Read the model definition and answer for the solid it produces. Units are mm, in the model's axes. Coordinates: 2 decimals unless noted, no trailing zeros. Loops run counter-clockwise (first coordinate to the right, second up) from the corner with the lowest first, then second, coordinate; pieces in that order, holes last.
Q1. Straight lines are drawn through the part: line 1 (X direction, y = 0.4, z = 0); line 2 (X direction, y = 0.3, z = -3); line 3 (Z direction, x = 2, y = 0.8). For each, find the intervals that lie inside material, in ascending order.
Q2. Section B-B (z = 3.75) is taken. Give the vertices of the cut face in (x, y), then the cut area to 3 significant figures.
Q3. A flat-ended cylindrical pin translates along its axis: P1, Ø0.7, axis at x = 0, z = 0, coming from the +Y side. Find the tip coordinate at first contact, or state that the pin passes through.
Q4. Section C-C (x = -3.75) is taken. Give the vertices of the cut face in (y, z).
Q5. Section D-D (y = 0.85) is taken. Count the separate pieces of the cut face and the enclosed holes in it, then the cut area to 3 significant figures.
Q6. Section A-A (x = 0) is taken. Give the vertices of the cut face in (y, z), then the cut area to 3 significant figures.
Q7. The mould has two halves that part along Z. Classify faces 1 (the face through (2.285, 0.493, -3.584)), 2 (the face through (0.525, 0.493, -0.165)), 3 (the face through (0, 1, 1)): pulls with the +Z half, pulls with the -Z half, needs draft (parallel to the pull), parting line crosses it, or undercut.
from build123d import *

# Parameters (mm, degrees)
ESQUISSE1_R        = 4.25
ESQUISSE1_R_2      = 0.55
ESQUISSE1_R_3      = 0.2
ESQUISSE1_R_4      = 0.3
BOSS_EXTRU_2_DEPTH = 1


with BuildPart() as part:
    # Esquisse1 → Boss.-Extru.2 (new body)
    with BuildSketch(Plane(origin=(0, 0, 0), x_dir=(1, 0, 0), z_dir=(0, 1, 0))):
        Circle(ESQUISSE1_R)
        Circle(ESQUISSE1_R_2, mode=Mode.SUBTRACT)
        with Locations((0, 3)):
            Circle(ESQUISSE1_R_3, mode=Mode.SUBTRACT)
        with Locations((0, 3.75)):
            Circle(ESQUISSE1_R_4, mode=Mode.SUBTRACT)
        with Locations((0.717946993, 2.912825452)):
            Circle(ESQUISSE1_R_3, mode=Mode.SUBTRACT)
        with Locations((1.394169516, 2.656368077)):
            Circle(ESQUISSE1_R_3, mode=Mode.SUBTRACT)
        with Locations((1.989367975, 2.245532245)):
            Circle(ESQUISSE1_R_3, mode=Mode.SUBTRACT)
        with Locations((2.468951598, 1.70419424)):
            Circle(ESQUISSE1_R_3, mode=Mode.SUBTRACT)
        with Locations((2.805048728, 1.063814661)):
            Circle(ESQUISSE1_R_3, mode=Mode.SUBTRACT)
        with Locations((2.978126622, 0.361610041)):
            Circle(ESQUISSE1_R_3, mode=Mode.SUBTRACT)
        with Locations((2.978126622, -0.361610041)):
            Circle(ESQUISSE1_R_3, mode=Mode.SUBTRACT)
        with Locations((2.805048728, -1.063814661)):
            Circle(ESQUISSE1_R_3, mode=Mode.SUBTRACT)
        with Locations((2.468951598, -1.70419424)):
            Circle(ESQUISSE1_R_3, mode=Mode.SUBTRACT)
        with Locations((1.989367975, -2.245532245)):
            Circle(ESQUISSE1_R_3, mode=Mode.SUBTRACT)
        with Locations((1.394169516, -2.656368077)):
            Circle(ESQUISSE1_R_3, mode=Mode.SUBTRACT)
        with Locations((0.717946993, -2.912825452)):
            Circle(ESQUISSE1_R_3, mode=Mode.SUBTRACT)
        with Locations((0, -3)):
            Circle(ESQUISSE1_R_3, mode=Mode.SUBTRACT)
        with Locations((-0.717946993, -2.912825452)):
            Circle(ESQUISSE1_R_3, mode=Mode.SUBTRACT)
        with Locations((-1.394169516, -2.656368077)):
            Circle(ESQUISSE1_R_3, mode=Mode.SUBTRACT)
        with Locations((-1.989367975, -2.245532245)):
            Circle(ESQUISSE1_R_3, mode=Mode.SUBTRACT)
        with Locations((-2.468951598, -1.70419424)):
            Circle(ESQUISSE1_R_3, mode=Mode.SUBTRACT)
        with Locations((-2.805048728, -1.063814661)):
            Circle(ESQUISSE1_R_3, mode=Mode.SUBTRACT)
        with Locations((-2.978126622, -0.361610041)):
            Circle(ESQUISSE1_R_3, mode=Mode.SUBTRACT)
        with Locations((-2.978126622, 0.361610041)):
            Circle(ESQUISSE1_R_3, mode=Mode.SUBTRACT)
        with Locations((-2.805048728, 1.063814661)):
            Circle(ESQUISSE1_R_3, mode=Mode.SUBTRACT)
        with Locations((-2.468951598, 1.70419424)):
            Circle(ESQUISSE1_R_3, mode=Mode.SUBTRACT)
        with Locations((-1.989367975, 2.245532245)):
            Circle(ESQUISSE1_R_3, mode=Mode.SUBTRACT)
        with Locations((-1.394169516, 2.656368077)):
            Circle(ESQUISSE1_R_3, mode=Mode.SUBTRACT)
        with Locations((-0.717946993, 2.912825452)):
            Circle(ESQUISSE1_R_3, mode=Mode.SUBTRACT)
        with Locations((3.75, 0)):
            Circle(ESQUISSE1_R_4, mode=Mode.SUBTRACT)
        with Locations((0, -3.75)):
            Circle(ESQUISSE1_R_4, mode=Mode.SUBTRACT)
        with Locations((-3.75, 0)):
            Circle(ESQUISSE1_R_4, mode=Mode.SUBTRACT)
    extrude(amount=BOSS_EXTRU_2_DEPTH)


solid = part.part
Numbers:
1. line 1: x = -4.25 to -4.05, -3.45 to -0.55, 0.55 to 3.45, 4.05 to 4.25
1. line 2: x = -3.01 to -0.9, -0.54 to -0.2, 0.2 to 0.54, 0.9 to 3.01
1. line 3: z = -3.75 to -2.45, -2.05 to 2.05, 2.45 to 3.75
2. outline: (-2, 0) - (-0.3, 0) - (-0.3, 1) - (-2, 1) - close; (0.3, 0) - (2, 0) - (2, 1) - (0.3, 1) - close
2. area: 3.40 mm2
3. P1: passes through
4. outline: (0, -2) - (1, -2) - (1, -0.3) - (0, -0.3) - close; (0, 0.3) - (1, 0.3) - (1, 2) - (0, 2) - close
5. separate pieces: 1
5. enclosed holes: 31
5. area: 51.4 mm2
6. outline: (0, -4.25) - (1, -4.25) - (1, -4.05) - (0, -4.05) - close; (0, -3.45) - (1, -3.45) - (1, -3.2) - (0, -3.2) - close; (0, -2.8) - (1, -2.8) - (1, -0.55) - (0, -0.55) - close; (0, 0.55) - (1, 0.55) - (1, 2.8) - (0, 2.8) - close; (0, 3.2) - (1, 3.2) - (1, 3.45) - (0, 3.45) - close; (0, 4.05) - (1, 4.05) - (1, 4.25) - (0, 4.25) - close
6. area: 5.40 mm2
7. face 1: parting line crosses it
7. face 2: undercut
7. face 3: needs draft
